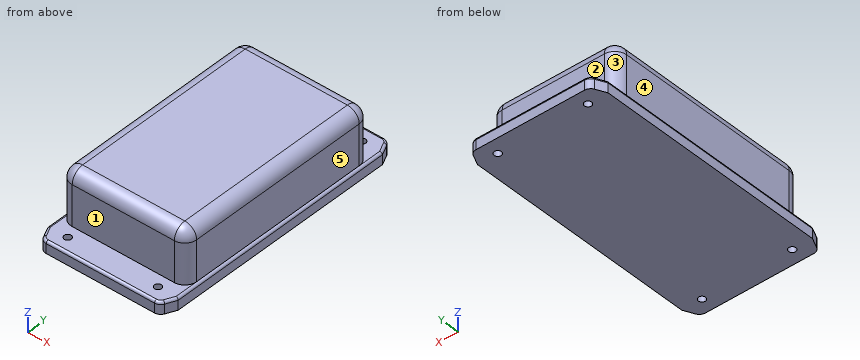
```python
from build123d import *

# Parameters (mm, degrees)
F1_DEPTH = 5
F2_W     = 53
F2_H     = 88
F3_DEPTH = 22
F4_R     = 1.5
F5_DEPTH = 25
F6_R     = 5
F7_R     = 0.99999


# Not quite as in the source:
# - a fillet or chamfer is up to 0.001 mm smaller than in the source, because OpenCascade refuses the exact size


with BuildPart() as f1:
    # F0 (on Top) → F1 (new body)
    with BuildSketch(Plane.XY):
        with BuildLine():
            Line((22.7909432686, 55), (-22.7909432686, 55))
            ThreePointArc((-22.7909432686, 55), (-24.4028420937, 54.5301743374), (-25.5098666298, 53.2678547852))
            Line((-25.5098666298, 53.2678547852), (-27.5, 49))
            Line((-27.5, 49), (-27.5, -49))
            Line((-27.5, -49), (-25.5098666298, -53.2678547852))
            ThreePointArc((-25.5098666298, -53.2678547852), (-24.4028420937, -54.5301743374), (-22.7909432686, -55))
            Line((-22.7909432686, -55), (22.7909432686, -55))
            ThreePointArc((22.7909432686, -55), (24.4028420937, -54.5301743374), (25.5098666298, -53.2678547852))
            Line((25.5098666298, -53.2678547852), (27.5, -49))
            Line((27.5, -49), (27.5, 49))
            Line((27.5, 49), (25.5098666298, 53.2678547852))
            ThreePointArc((25.5098666298, 53.2678547852), (24.4028420937, 54.5301743374), (22.7909432686, 55))
        make_face()
    extrude(amount=F1_DEPTH)

    # F2 (on face) → F3 (join)
    with BuildSketch(Plane.XY.offset(5)):
        Rectangle(F2_W, F2_H)
    extrude(amount=F3_DEPTH)

    # F4 (on face) → F5 (cut)
    with BuildSketch(Plane.XY.offset(5)):
        with Locations((-19, 49)):
            Circle(F4_R)
        with Locations((19, 49)):
            Circle(F4_R)
        with Locations((-19, -49)):
            Circle(F4_R)
        with Locations((19, -49)):
            Circle(F4_R)
    extrude(amount=-F5_DEPTH, mode=Mode.SUBTRACT)

    # F6
    f6_edges = [f1.edges().sort_by_distance(p)[0] for p in [
        (-26.5, 0, 27),
        (0, 44, 27),
        (26.5, 0, 27),
        (0, -44, 27),
        (26.5, -44, 16),
        (26.5, 44, 16),
        (-26.5, 44, 16),
        (-26.5, -44, 16),
    ]]
    fillet(f6_edges, radius=F6_R)

    # F7 (radius 1 in the source; OpenCascade refuses exactly that, so slightly less here)
    f7_edges = [f1.edges().sort_by_distance(p)[0] for p in [
        (27.5, 0, 5),
        (26.504933, -51.133927, 5),
        (26.504933, 51.133927, 5),
        (-27.5, 0, 5),
    ]]
    fillet(f7_edges, radius=F7_R)


solid = f1.part
```
Read the model definition and answer for the solid it produces. Units are mm, in the model's axes. Face numbers are marked on the shaded views. A direction names the side the tool comes from. Coordinates: 2 decimals unless noted, no trailing zeros. Write each loop counter-clockwise with the first axis right and the second up, starting at its lowest first coordinate (ties: lowest second). Pieces come first, ordered by that corner, then holes. Notation, with made-up numbers: (-27, 53) -> (25, 53) arc R23 cw to (25, 77) -> close; hole circle Ø7 at (38, 66.5). An arc over 180 degrees is marked (long way). Return JSON: item names as keys, results as strings.
1. Each of these flat-tipped pins is pushed along its axis until it touches: P1, Ø5, axis at x = -14.5, z = 9, coming from the -Y side; P2, Ø6, axis at y = -34.5, z = 18.5, coming from the -X side; P3, Ø6, axis at x = 7, z = 17, coming from the +Y side. Where does it stop, or does it pass through?
Found:
{"P1": "y = -44", "P2": "x = -26.5", "P3": "y = 44"}
2. A cutting plane is placed at B-B (z = 10). Determine the outline of the cut face in (x, y), and give its area (3 significant figures).
Found:
{"outline": "(-26.5, -39) arc R5 ccw to (-21.5, -44) -> (21.5, -44) arc R5 ccw to (26.5, -39) -> (26.5, 39) arc R5 ccw to (21.5, 44) -> (-21.5, 44) arc R5 ccw to (-26.5, 39) -> close", "area": "4,640 mm2"}
3. A cutting plane is placed at A-A (x = 19). Determine the outline of the cut face in (y, z), and give its area (3 significant figures).
Found:
{"outline": "(-55, 0) -> (-50.5, 0) -> (-50.5, 5) -> (-54, 5) arc R1 ccw to (-55, 4) -> close; (-47.5, 0) -> (47.5, 0) -> (47.5, 5) -> (44, 5) -> (44, 22) arc R5 ccw to (39, 27) -> (-39, 27) arc R5 ccw to (-44, 22) -> (-44, 5) -> (-47.5, 5) -> close; (50.5, 0) -> (55, 0) -> (55, 4) arc R1 ccw to (54, 5) -> (50.5, 5) -> close", "area": "2,440 mm2"}
4. A cutting plane is placed at D-D (x = 4). Determine the outline of the cut face in (y, z), and give its area (3 significant figures).
Found:
{"outline": "(-55, 0) -> (55, 0) -> (55, 4) arc R1 ccw to (54, 5) -> (44, 5) -> (44, 22) arc R5 ccw to (39, 27) -> (-39, 27) arc R5 ccw to (-44, 22) -> (-44, 5) -> (-54, 5) arc R1 ccw to (-55, 4) -> close", "area": "2,470 mm2"}
5. Find the intervals of material crossed by line 1 along Y through (x, z) = (-19, 2.75); line 2 along Z through (x, y) = (16, 49.5); line 3 along X through (y, z) = (1, 6.75), in increasing order. Write a range as from..to.
Found:
{"line 1": "-55..-50.5, -47.5..47.5, 50.5..55", "line 2": "0..5", "line 3": "-26.5..26.5"}
6. A tool of negligible diameter and unlimited length cuts with its end or side. For the marked faces 1, 2, 3, 4 and 5, from which of +Z, -Z, +X, -X, +Y, -Y can it reach the whole face along a straight path? Write none if from no direction.
Found:
{"face 1": "+Z, +X, -X, -Y", "face 2": "+Z, +X, -X, +Y", "face 3": "+Z, -X, +Y", "face 4": "+Z, -X, +Y, -Y", "face 5": "+Z, +X, +Y, -Y"}
